Can you work these out from the model? Positions are in its coordinate system, mm. A direction names the side the tool comes from. Coordinates: 2 decimals unless noted, no trailing zeros. Order: outer loops, then holes, each group sorted by start corner. A loop starts at its lowest first (then second) coordinate and runs counter-clockwise, first axis right, second up. Notation, with made-up numbers: (20.25, 73.25) -> (76.25, 73.25) arc R32 cw to (76.25, 109.25) -> close; hole circle Ø5 at (82, 62). An arc over 180 degrees is marked (long way). Answer as a JSON object with one key per item and string values. Group by question number.
(1) I want a section at D-D, the plane y = -1. List the corners of the cut face in (x, z) for me.
(2) I want a section at A-A, the plane x = 0. List the corners of the cut face in (y, z) for me.
(3) For pin 1 (2 mm diameter, centred on x = -1.5, y = 3, fed in from +Z); pin 2 (4 mm diameter, centred on y = 3, z = 0, fed in from +X); pin 3 (1 mm diameter, centred on y = 4, z = 3, fed in from +X); pin 4 (5 mm diameter, centred on x = 2.5, z = -4, fed in from +Y), each with a flat end and sliding along its axis, tell me the tip position at first contact or that it passes through.
(4) Which directions (+Z, -Z, +X, -X, +Y, -Y) give clear straight access to the entire face, cutting with the end or side of a thin tool? Please do faces 1 (the cylindrical face through (-1.978, 4.93, -2.579)), 2 (the cylindrical face through (-0.488, -0.986, -0.108)).
(5) I want a section at B-B, the plane y = 1.25. List the corners of the cut face in (x, z) for me.
(6) I want a section at C-C, the plane y = 7.75. List the corners of the cut face in (x, z) for me, plus the area to 3 significant figures.
(7) If we mould it in two halves opening along X, with no side actions, what happens to faces 3 (the cylindrical face through (-3.417, 4.93, -0.759)), 4 (the flat face through (1, -2, 0)), 5 (the cylindrical face through (0.225, 0.986, 0.715))? For each: pulls with the +X half, pulls with the -X half, needs draft (parallel to the pull), parting line crosses it, or undercut.
(8) I need wall thicknesses on line 1 (X direction, y = 0.5, z = 0); line 2 (X direction, y = 4, z = 0); line 3 (Y direction, x = 1.25, z = 4). Which ranges of each line are inside material? Lowest first, please.
from build123d import *

# Parameters (mm, degrees)
SKETCH2_R           = 5
SKETCH1_R           = 5.5
SKETCH3_R           = 0.5
CUT_EXTRUDE1_DEPTH  = 9.031189364
SKETCH4_R           = 3.5
SKETCH4_R_2         = 3.25
BOSS_EXTRUDE1_DEPTH = 10
SKETCH5_R           = 0.75
SKETCH5_R_2         = 0.25
BOSS_EXTRUDE2_DEPTH = 2


with BuildPart() as part:
    # Sketch2 → Loft1 section 0
    with BuildSketch(Plane(origin=(0, -2, 0), x_dir=(1, 0, 0), z_dir=(0, 1, 0))):
        Circle(SKETCH2_R)
    # Sketch1 → Loft1 section 1
    with BuildSketch(Plane(origin=(0, 0, 0), x_dir=(1, 0, 0), z_dir=(0, 1, 0))):
        Circle(SKETCH1_R)
    loft()

    # Sketch3 → Cut-Extrude1 (cut, through all)
    with BuildSketch(Plane(origin=(0, 0, 0), x_dir=(1, 0, 0), z_dir=(0, 1, 0))):
        with Locations(Location((0, 0, 0), (0, 0, 270))):
            Circle(SKETCH3_R)
    extrude(amount=-CUT_EXTRUDE1_DEPTH, mode=Mode.SUBTRACT)

    # Sketch4 → Boss-Extrude1 (add)
    with BuildSketch(Plane(origin=(0, 0, 0), x_dir=(1, 0, 0), z_dir=(0, 1, 0))):
        with Locations(Location((0, 0, 0), (0, 0, 270))):
            Circle(SKETCH4_R)
        with Locations(Location((0, 0, 0), (0, 0, 270))):
            Circle(SKETCH4_R_2, mode=Mode.SUBTRACT)
    extrude(amount=BOSS_EXTRUDE1_DEPTH)

    # Sketch5 → Boss-Extrude2 (add)
    with BuildSketch(Plane(origin=(0, 0, 0), x_dir=(1, 0, 0), z_dir=(0, 1, 0))):
        with Locations(Location((0, 0, 0), (0, 0, 270))):
            Circle(SKETCH5_R)
        with Locations(Location((0, 0, 0), (0, 0, 270))):
            Circle(SKETCH5_R_2, mode=Mode.SUBTRACT)
    extrude(amount=BOSS_EXTRUDE2_DEPTH)


solid = part.part
Computed values:
{
 "1": {"outline": "circle Ø10.5 at (0, 0); hole circle Ø1 at (0, 0)"},
 "2": {"outline": "(-2, -5) -> (0, -5.5) -> (0, -3.5) -> (10, -3.5) -> (10, -3.25) -> (0, -3.25) -> (0, -0.75) -> (2, -0.75) -> (2, -0.25) -> (0, -0.25) -> (0, -0.5) -> (-2, -0.5) -> close; (-2, 0.5) -> (0, 0.5) -> (0, 0.25) -> (2, 0.25) -> (2, 0.75) -> (0, 0.75) -> (0, 3.25) -> (10, 3.25) -> (10, 3.5) -> (0, 3.5) -> (0, 5.5) -> (-2, 5) -> close"},
 "3": {"pin 1": "stops at z = 3.46", "pin 2": "stops at x = 3.5", "pin 3": "stops at x = 2.45", "pin 4": "stops at y = 10"},
 "4": {"face 1": "+Y", "face 2": "-Y"},
 "5": {"outline": "circle Ø7 at (0, 0); circle Ø1.5 at (0, 0); hole circle Ø6.5 at (0, 0); hole circle Ø0.5 at (0, 0)"},
 "6": {"outline": "circle Ø7 at (0, 0); hole circle Ø6.5 at (0, 0)", "area": "5.30 mm2"},
 "7": {"face 3": "parting line crosses it", "face 4": "needs draft", "face 5": "undercut"},
 "8": {"line 1": "x = -3.5 to -3.25, -0.75 to -0.25, 0.25 to 0.75, 3.25 to 3.5", "line 2": "x = -3.5 to -3.25, 3.25 to 3.5", "line 3": "y = -2 to 0"}
}
